Study the drawing (mm; zero at the part's minimum x, y, z) and answer. Coordinates: 2 decimals unless noted, no trailing zeros. Order: outer loops, then holes, each group sorted by start corner. A loop starts at its lowest first (then second) coordinate and runs counter-clockwise, first axis right, second up. Notation, with made-up numbers: (88.5, 74.5) -> (138.5, 74.5) arc R23 cw to (138.5, 88.5) -> close; hole circle Ø1 at (15, 37). An arc over 180 degrees is marked (long way). Answer in a Markdown table with one row per item. Add a question column.
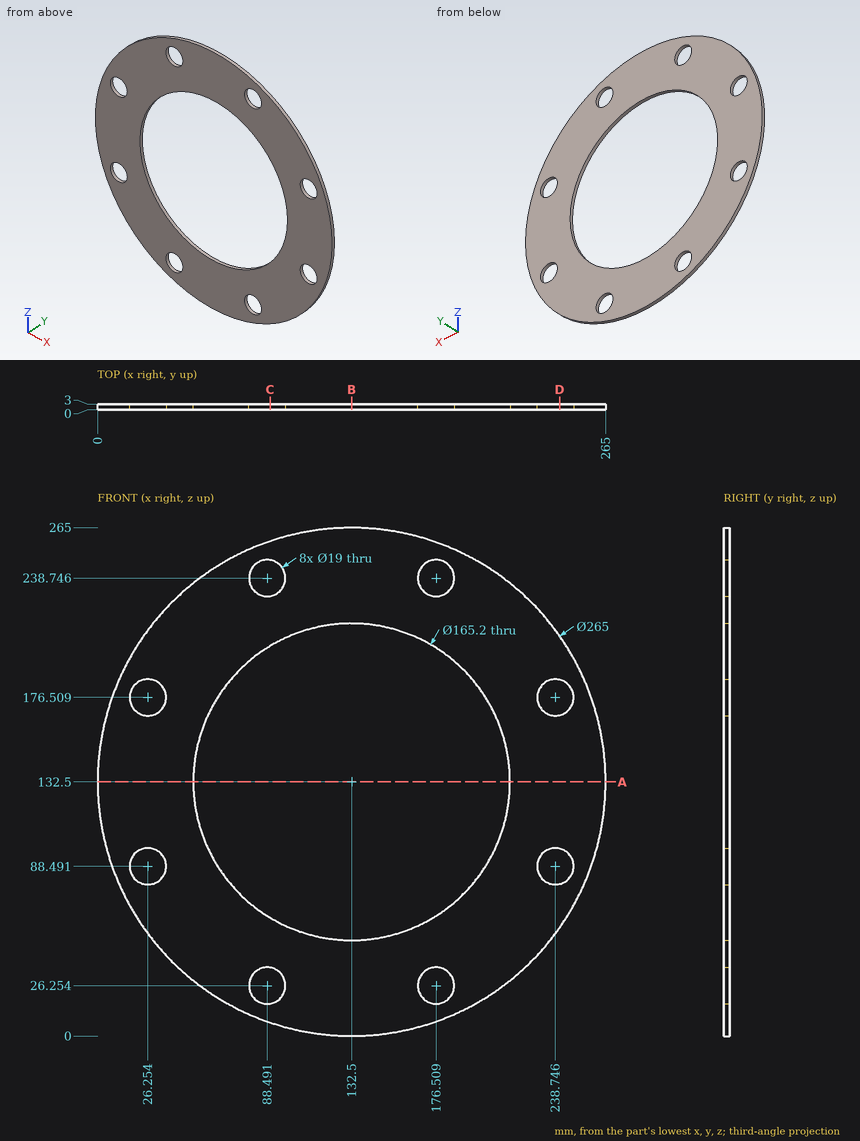
Q1. Given pin 1 (15 mm diameter, centred on x = 238.75, z = 88.49, fed in from -Y); pin 2 (1.5 mm diameter, centred on y = 1, z = 103, fed in from -X), each flat-ended and moving along its own axis, determine where each tip first touches the part or whether it passes through.
Q2. A cutting plane is placed at A-A (z = 132.5). Determine the outline of the cut face in (x, y).
Q3. Straight lines are drawn through the part: line 1 (X direction, y = 1.7, z = 243) (1 decimal); line 2 (X direction, y = 1.45, z = 180.5) (1 decimal); line 3 (X direction, y = 1.65, z = 246) (1 decimal). For each, find the intervals that lie inside material, in ascending order.
Q4. A cutting plane is placed at D-D (x = 241). Determine the outline of the cut face in (y, z).
Q5. A cutting plane is placed at B-B (x = 132.5). Determine the outline of the cut face in (y, z).
Q6. A cutting plane is placed at C-C (x = 90). Determine the outline of the cut face in (y, z) (1 decimal).
Returned:
| question | item | result |
|---|---|---|
| 1 | pin 1 | passes through |
| 1 | pin 2 | stops at x = 3.16 |
| 2 | outline | (0, 0) -> (49.9, 0) -> (49.9, 3) -> (0, 3) -> close; (215.1, 0) -> (265, 0) -> (265, 3) -> (215.1, 3) -> close |
| 3 | line 1 | x = 59.4 to 80, 97 to 168, 185 to 205.6 |
| 3 | line 2 | x = 9 to 17.6, 34.9 to 65.3, 199.7 to 230.1, 247.4 to 256 |
| 3 | line 3 | x = 64.1 to 82.4, 94.6 to 170.4, 182.6 to 200.9 |
| 4 | outline | (0, 56.45) -> (3, 56.45) -> (3, 79.26) -> (0, 79.26) -> close; (0, 97.72) -> (3, 97.72) -> (3, 167.28) -> (0, 167.28) -> close; (0, 185.74) -> (3, 185.74) -> (3, 208.55) -> (0, 208.55) -> close |
| 5 | outline | (0, 0) -> (3, 0) -> (3, 49.9) -> (0, 49.9) -> close; (0, 215.1) -> (3, 215.1) -> (3, 265) -> (0, 265) -> close |
| 6 | outline | (0, 7) -> (3, 7) -> (3, 16.9) -> (0, 16.9) -> close; (0, 35.6) -> (3, 35.6) -> (3, 61.7) -> (0, 61.7) -> close; (0, 203.3) -> (3, 203.3) -> (3, 229.4) -> (0, 229.4) -> close; (0, 248.1) -> (3, 248.1) -> (3, 258) -> (0, 258) -> close |
